Design review of the part shown in the three views and the two pictorial views. Dimensions are in mm from the part's minimum x, y and z. Round coordinates to 2 decimals unless told otherwise and drop trailing zeros. Loops run counter-clockwise (first coordinate to the right, second up) from the corner with the lowest first, then second, coordinate; pieces in that order, holes last. Notation, with made-up numbers: (7.5, 17.25) -> (31.5, 17.25) arc R18 ccw to (31.5, 44.25) -> close; hole circle Ø1 at (79, -24.75). An arc over 180 degrees is marked (long way). Write each question's results on one line, items separated by ' | '. Start each with the question number.
Item 1: For L1, parallel to X at y = 3.5, z = 34.5; L2, parallel to Y at x = 2.5, z = 18.5 (1 decimal), list the stretches that pass through material, from the lowest coordinate up. Write a range as from..to.
Item 2: Clearance check with a flat-ended pin moving along its axis: pin 1 Ø4 at (y, z) = (5.5, 28.5) entering from -X. State where the tip first meets the part, or that it passes through.
Item 3: We need section A-A (y = 3.5). Give the boundary of the cut face in (x, z).
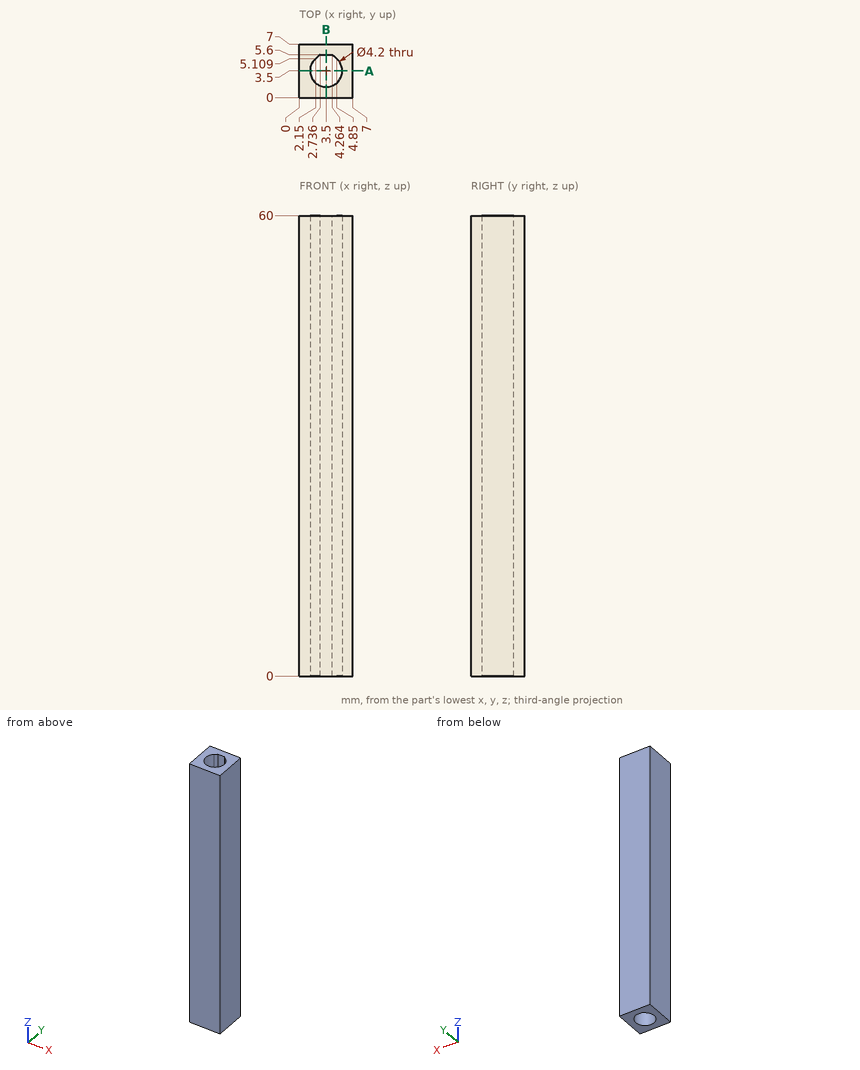
Here are the results:
1) L1: x = 0..1.4, 5.6..7 | L2: y = 0..1.7, 5.4..7
2) pin 1: stops at x = 0
3) outline: (0, 0) -> (1.4, 0) -> (1.4, 60) -> (0, 60) -> close; (5.6, 0) -> (7, 0) -> (7, 60) -> (5.6, 60) -> close
